Here's how the part is built. I have some questions about the finished solid (model axes, mm). Face numbers are marked on the shaded views. A direction names the side the tool comes from. Coordinates: 2 decimals unless noted, no trailing zeros. Loops run counter-clockwise (first coordinate to the right, second up) from the corner with the lowest first, then second, coordinate; pieces in that order, holes last.
from build123d import *

# Parameters (mm, degrees)
SKETCH2_R           = 0.75
BOSS_EXTRUDE1_DEPTH = 1
FILLET1_R           = 0.7
SKETCH3_R           = 2
BOSS_EXTRUDE2_DEPTH = 5
SKETCH4_R           = 6
BOSS_EXTRUDE3_DEPTH = 1


with BuildPart() as part:
    # Sketch1 → Revolve1 (revolve)
    with BuildSketch(Plane(origin=(0, 0, 0), x_dir=(1, 0, 0), z_dir=(0, 1, 0)), mode=Mode.PRIVATE) as revolve1_sk:
        Polygon((0, 31.22), (0, 0), (1, -1.528489116), (1, -7.748489116), (6, -7.748489116), (6, 31.22), align=None)
    revolve(revolve1_sk.sketch.rotate(Axis((6, 0, 7.748489116), (0, 0, -1)), 180), axis=Axis((6, 0, 7.748489116), (0, 0, -1)))

    # Sketch2 → Boss-Extrude1 (add)
    with BuildSketch(Plane.XY.offset(7.748489116)):
        with Locations(Location((9.311049148, 0, 0), (0, 0, 180))):
            Circle(SKETCH2_R)
    extrude(amount=BOSS_EXTRUDE1_DEPTH)

    # Fillet1
    fillet1_edges = [part.edges().sort_by_distance(p)[0] for p in [
        (10.061049148, 0, 8.748489116),
    ]]
    fillet(fillet1_edges, radius=FILLET1_R)

    # Sketch3 → Boss-Extrude2 (add)
    with BuildSketch(Plane.XY.offset(7.748489116)):
        with Locations(Location((3.423004201, 0, 0), (0, 0, 180))):
            Circle(SKETCH3_R)
    extrude(amount=BOSS_EXTRUDE2_DEPTH)

    # Sketch4 → Boss-Extrude3 (add)
    with BuildSketch(Plane(origin=(0, 0, -31.22), x_dir=(-1, 0, 0), z_dir=(0, 0, -1))):
        with Locations((-5.996963967, 0)):
            Circle(SKETCH4_R)
    extrude(amount=BOSS_EXTRUDE3_DEPTH)


solid = part.part
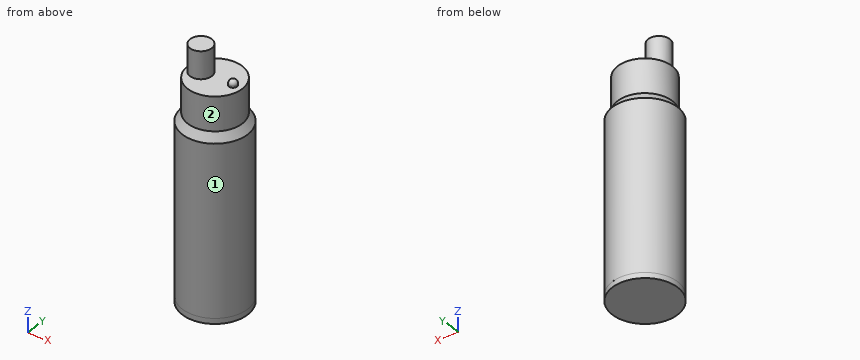
Q1. Suppose I cut it at B-B on z = 4. Write out the boundary of the cut face in (x, y), and give its area (3 significant figures).
Q2. Will these pins go through, and if not, where does the flat tip stop? P1, Ø5, axis at y = 2.5, z = -14, coming from the +X side; P2, Ø1.5, axis at x = 2.5, z = -4.5, coming from the -Y side; P3, Ø3, axis at y = 3, z = -18, coming from the +X side; P4, Ø1.5, axis at x = 3, z = -16, coming from the +Y side.
Q3. Please list where these lines run through material, in increasing order: probe 1 along Z at (x, y) = (1.75, 1.5); probe 2 along X at (y, z) = (0.25, -11); probe 3 along X at (y, z) = (4.25, -23).
Q4. For the marked faces 1 and 2, which set-ups out of +Z, -Z, +X, -X, +Y, -Y let a thin tool reach every point of the face, with its end or its side?
Q5. Suppose I cut it at A-A on z = -28. Write out the boundary of the cut face in (x, y), and give its area (3 significant figures).
Check values:
1. outline: circle Ø10 at (6, 0)
1. area: 78.5 mm2
2. P1: stops at x = 12
2. P2: stops at y = -5.33
2. P3: stops at x = 11.81
2. P4: stops at y = 5.56
3. probe 1: z = -32.22 to 7.75
3. probe 2: x = 0.01 to 11.99
3. probe 3: x = 1.76 to 10.24
4. face 1: +Z, -Z
4. face 2: +Z
5. outline: circle Ø12 at (6, 0)
5. area: 113 mm2
